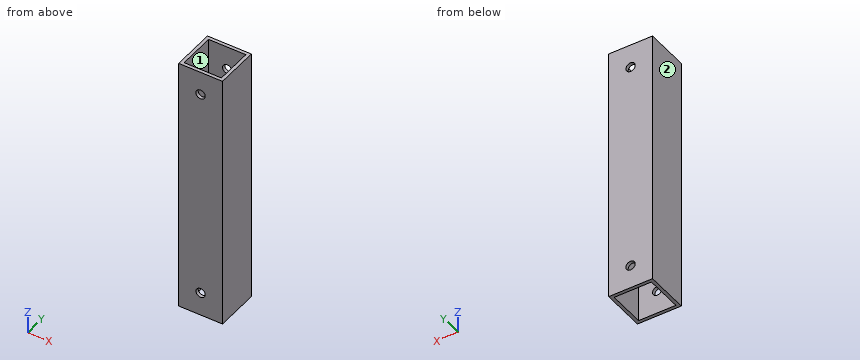
```python
from build123d import *

# Parameters (mm, degrees)
SKETCH1_W           = 20
SKETCH1_H           = 20
SKETCH1_W_2         = 17
SKETCH1_H_2         = 17
BOSS_EXTRUDE1_DEPTH = 118.4
SKETCH2_R           = 2.125
CUT_EXTRUDE1_DEPTH  = 121.492987348


with BuildPart() as part:
    # Sketch1 → Boss-Extrude1 (new body)
    with BuildSketch(Plane.XY):
        Rectangle(SKETCH1_W, SKETCH1_H)
        Rectangle(SKETCH1_W_2, SKETCH1_H_2, mode=Mode.SUBTRACT)
    extrude(amount=-BOSS_EXTRUDE1_DEPTH)

    # Sketch2 → Cut-Extrude1 (cut, through all)
    with BuildSketch(Plane(origin=(0, 10, 0), x_dir=(1, 0, 0), z_dir=(0, 1, 0))):
        with Locations(Location((0, 10.8, 0), (0, 0, 270))):
            Circle(SKETCH2_R)
        with Locations(Location((0, 107.6, 0), (0, 0, 90))):
            Circle(SKETCH2_R)
    extrude(amount=-CUT_EXTRUDE1_DEPTH, mode=Mode.SUBTRACT)


solid = part.part
```
Read the model definition and answer for the solid it produces. Units are mm, in the model's axes. Face numbers are marked on the shaded views. A direction names the side the tool comes from. Coordinates: 2 decimals unless noted, no trailing zeros. Write each loop counter-clockwise with the first axis right and the second up, starting at its lowest first coordinate (ties: lowest second). Pieces come first, ordered by that corner, then holes. Notation, with made-up numbers: (83, -4.5) -> (91, -4.5) arc R16 ccw to (91, 26.5) -> close; hole circle Ø3 at (2.25, 71.25). An arc over 180 degrees is marked (long way). Answer as a JSON object with one key per item and string values.
Q1. The part is cut by section A-A on y = 2.25. Give the vertices of the cut face in (x, z), then the cut area to 3 significant figures.
The answers:
{"outline": "(-10, -118.4) -> (-8.5, -118.4) -> (-8.5, 0) -> (-10, 0) -> close; (8.5, -118.4) -> (10, -118.4) -> (10, 0) -> (8.5, 0) -> close", "area": "355 mm2"}
Q2. The part is cut by section B-B on z = -30.5. Give the vertices of the cut face in (x, y).
The answers:
{"outline": "(-10, -10) -> (10, -10) -> (10, 10) -> (-10, 10) -> close; hole (-8.5, -8.5) -> (8.5, -8.5) -> (8.5, 8.5) -> (-8.5, 8.5) -> close"}
Q3. A flat-ended cylindrical pin translates along its axis: pin 1 Ø10 at (x, y) = (0, 2) entering from -Z. Find the tip coordinate at first contact, or state that the pin passes through.
The answers:
{"pin 1": "passes through"}
Q4. Consider line 1 (X direction, y = 3.75, z = -59.5); line 2 (X direction, y = 9, z = -107.6) (3 decimals). Determine where each line is inside the solid, lowest interval first. Write a range as [from, to].
The answers:
{"line 1": "x = [-10, -8.5], [8.5, 10]", "line 2": "x = [-10, -2.125], [2.125, 10]"}
Q5. The part is cut by section D-D on x = 0. Give the vertices of the cut face in (y, z) (3 decimals).
The answers:
{"outline": "(-10, -118.4) -> (-8.5, -118.4) -> (-8.5, -109.725) -> (-10, -109.725) -> close; (-10, -105.475) -> (-8.5, -105.475) -> (-8.5, -12.925) -> (-10, -12.925) -> close; (-10, -8.675) -> (-8.5, -8.675) -> (-8.5, 0) -> (-10, 0) -> close; (8.5, -118.4) -> (10, -118.4) -> (10, -109.725) -> (8.5, -109.725) -> close; (8.5, -105.475) -> (10, -105.475) -> (10, -12.925) -> (8.5, -12.925) -> close; (8.5, -8.675) -> (10, -8.675) -> (10, 0) -> (8.5, 0) -> close"}
Q6. A tool of negligible diameter and unlimited length cuts with its end or side. For the marked faces 1 and 2, from which of +Z, -Z, +X, -X, +Y, -Y can it reach the whole face along a straight path? Write none if from no direction.
The answers:
{"face 1": "+Z, -Z", "face 2": "+Z, -Z, -X, +Y, -Y"}
